Can you work these out from the model? Positions are in its coordinate system, mm. A direction names the side the tool comes from. Coordinates: 2 decimals unless noted, no trailing zeros. Loops run counter-clockwise (first coordinate to the right, second up) from the corner with the lowest first, then second, coordinate; pieces in that order, holes last.
Autodesk Inventor part; units mm, degrees
ref_plane "YZ Plane" through (0, 0, 0) normal (1, 0, 0) x (0, 1, 0)
ref_plane "XZ Plane" through (0, 0, 0) normal (0, 1, 0) x (-1, 0, 0)
ref_plane "XY Plane" through (0, 0, 0) normal (0, 0, 1) x (1, 0, 0)
sketch "Sketch1" plane through (0, 0, 0) normal (0, 1, 0) x (-1, 0, 0)
  line L0 (10, 12.5) -> (-10, 12.5)
  line L1 (-10, 12.5) -> (-10, -12.5)
  line L2 (-10, -12.5) -> (10, -12.5)
  line L3 (10, -12.5) -> (10, 12.5)
  line L4 (10, 0) -> (-10, 0) construction
  line L5 (0, 12.5) -> (0, -12.5) construction
  line L6 (10, 12.5) -> (8, 12.5)
  line L7 (8, 12.5) -> (8, -12.5)
  line L8 (8, -12.5) -> (10, -12.5)
  line L9 (10, -12.5) -> (10, 12.5)
  circle A0 centre (0, 6) radius 1.5
  circle A1 centre (0, 6) radius 2.75
  circle A2 centre (0, -6) radius 1.5
  circle A3 centre (0, -6) radius 2.75
  point P0 (0, 0)
  point P1 (0, 0)
  dimension "d0" = 20
  dimension "d1" = 25
  dimension "d2" = 2
  dimension "d3" = 3
  dimension "d4" = 5.5
  dimension "d5" = 6
extrude "Extrusion1" add sketch "Sketch1" along normal blind 2 contours L7 L2 L1 L0
extrude "Extrusion2" add sketch "Sketch1" along normal blind 1 contours A1 | A3
extrude "Extrusion3" add sketch "Sketch1" along normal blind 27 contours L3 L2 L7 L0
sketch "Sketch2" plane through (-8, 2, -12.5) normal (1, 0, 0) x (0, 0, -1)
  circle A0 centre (-12.5, 12.5) radius 12.5
  line L0 (-25, 25) -> (0, 25)
  line L1 (-12.5, 25) -> (-25, 25)
  line L2 (-25, 25) -> (-25, 12.5)
  line L3 (-25, 0) -> (-25, 25)
  line L4 (-12.5, 25) -> (0, 25)
  line L5 (0, 25) -> (0, 12.5)
  line L6 (0, 0) -> (0, 25)
  point P0 (-12.5, -2)
  point P1 (-25, 12.5)
  dimension "d12" = 25
extrude "Extrusion4" cut sketch "Sketch2" against normal blind 2 contours A0 L0 L5 | A0 L2 L0
sketch "Sketch3" plane through (-10, 0, -12.5) normal (-1, 0, 0) x (0, 0, 1)
  arc A0 (25, 14.5) -> (0, 14.5) centre (12.5, 14.5) ccw
  circle A1 centre (21, 14.5) radius 1.5
  circle A2 centre (21, 14.5) radius 2.75
  line L0 (12.5, 14.5) -> (12.5, 17.4625)
  circle A3 centre (4, 14.5) radius 1.5
  circle A4 centre (4, 14.5) radius 2.75
  circle A5 centre (12.5, 14.5) radius 3.5
  circle A6 centre (12.5, 6) radius 1.5
  circle A7 centre (12.5, 6) radius 2.75
  circle A8 centre (12.5, 23) radius 1.5
  circle A9 centre (12.5, 23) radius 2.75
  point P0 (12.5, 0)
  dimension "d15" = 3
  dimension "d16" = 5.5
  dimension "d17" = 8.5
  dimension "d22" = 7
  dimension "d25" = 3
  dimension "d26" = 5.5
  dimension "d27" = 8.5
  dimension "d28" = 3
  dimension "d29" = 5.5
  dimension "d30" = 8.5
extrude "Extrusion5" cut sketch "Sketch3" against normal blind 2 contours A1 | A3 | A6 | A8
extrude "Extrusion6" cut sketch "Sketch3" against normal blind 1 contours A2 | A4 | A7 | A9
extrude "Extrusion7" cut sketch "Sketch3" against normal blind 2 contours A5
properties part number "Bracket Motor JGA Depan_3DPrint"
Item 1: We'd pull the mould along X, two halves only. Please class faces 1 (the face through (0.596, 1.493, -3.315)), 2 (the face through (-9, 27, 0)), 3 (the face through (-10, 10, 0)): +X half, -X half, draft (parallel to the pull), parting line (faces both ways), or undercut.
Results are:
face 1: undercut
face 2: draft
face 3: -X half
Item 2: Suppose I cut it at D-D, the plane x = 3.5. Please give me the cut outline in (y, z).
Results are:
outline: (0, -12.5) - (2, -12.5) - (2, 12.5) - (0, 12.5) - close
Item 3: Suppose I cut it at C-C, the plane z = -5. Please give me the cut outline in (x, y), plus the area to 3 significant figures.
Results are:
outline: (-10, 0) - (-1.12, 0) - (-1.12, 1) - (-2.56, 1) - (-2.56, 2) - (-8, 2) - (-8, 25.96) - (-10, 25.96) - close; (1.12, 0) - (10, 0) - (10, 2) - (2.56, 2) - (2.56, 1) - (1.12, 1) - close
area: 80.6 mm2
Item 4: I'm going to push flat-ended pins straight in: P1, Ø3, axis at y = 15, z = -9, coming from the -X side; P2, Ø7, axis at y = 14.5, z = 8.5, coming from the -X side; P3, Ø6.5, axis at y = 23, z = 0, coming from the +X side; P4, Ø5, axis at x = 0, z = -6, coming from the +Y side. Where does each tip first touch, or does it pass through?
Results are:
P1: stops at x = -9
P2: stops at x = -10
P3: stops at x = -8
P4: stops at y = 1
Item 5: I need wall thicknesses on line 1 along Z through (x, y) = (0, 0.75); line 2 along Z through (x, y) = (0, 1.3); line 3 along Y through (x, z) = (-8.7, 0). Which ranges of each line are inside material? Lowest first, please.
Results are:
line 1: z = -12.5 to -7.5, -4.5 to 4.5, 7.5 to 12.5
line 2: z = -12.5 to -8.75, -3.25 to 3.25, 8.75 to 12.5
line 3: y = 0 to 4.5, 7.5 to 11, 18 to 21.5, 24.5 to 27
Item 6: On a 3-axis mill with a long thin cutter (end or side, diameter ignored), from which of +Z, -Z, +X, -X, +Y, -Y can I reach the whole of each face in a straight line? I mean faces 4 (the face through (-9.507, 17.227, 8.142)), 5 (the face through (-1.2, 1, -7.2)), 6 (the face through (-8, 12, -3)). Say none if no direction works.
Results are:
face 4: -X
face 5: +Y
face 6: +Z, -Z, +X, +Y
Item 7: Suppose I cut it at A-A, the plane y = 6. Please give me the cut outline in (x, z).
Results are:
outline: (-10, -12.5) - (-8, -12.5) - (-8, -1.5) - (-9, -1.5) - (-9, -2.75) - (-10, -2.75) - close; (-10, 2.75) - (-9, 2.75) - (-9, 1.5) - (-8, 1.5) - (-8, 12.5) - (-10, 12.5) - close
Item 8: Suppose I cut it at B-B, the plane x = 0. Please give me the cut outline in (y, z).
Results are:
outline: (0, -12.5) - (2, -12.5) - (2, -8.75) - (1, -8.75) - (1, -7.5) - (0, -7.5) - close; (0, -4.5) - (1, -4.5) - (1, -3.25) - (2, -3.25) - (2, 3.25) - (1, 3.25) - (1, 4.5) - (0, 4.5) - close; (0, 7.5) - (1, 7.5) - (1, 8.75) - (2, 8.75) - (2, 12.5) - (0, 12.5) - close
